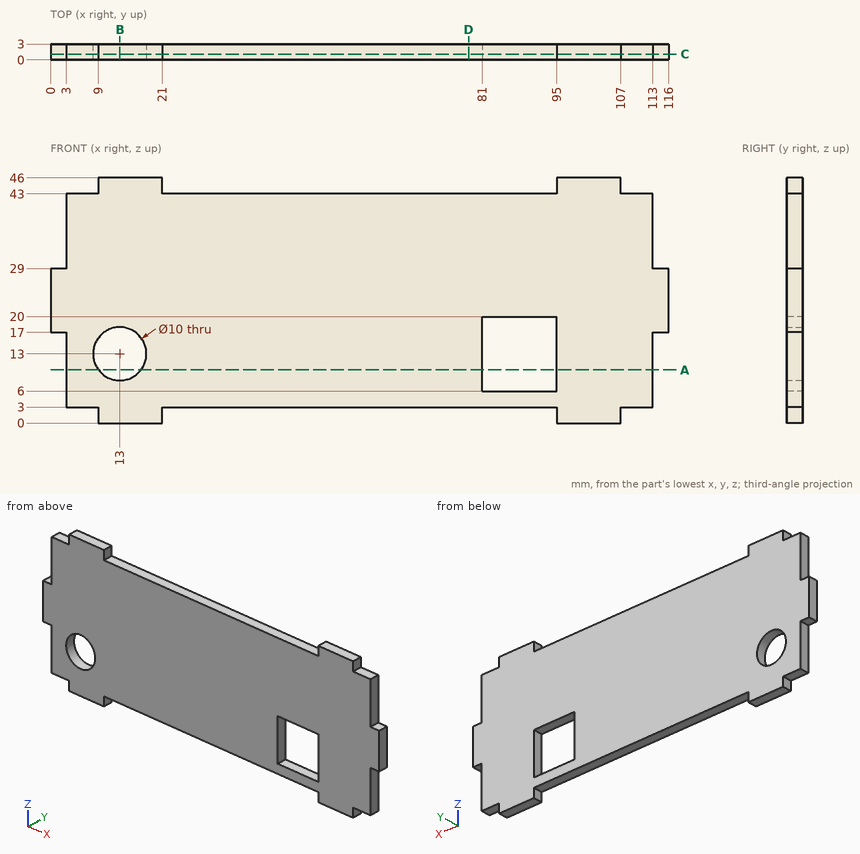
Can you work these out from the drawing? Everything is in mm from the part's minimum corner. Coordinates: 2 decimals unless noted, no trailing zeros. Loops run counter-clockwise (first coordinate to the right, second up) from the corner with the lowest first, then second, coordinate; pieces in that order, holes last. Notation, with made-up numbers: (3, 76.25) -> (10, 76.25) arc R31 ccw to (10, 101.25) -> close; hole circle Ø1 at (24, 83.5). An arc over 180 degrees is marked (long way). Return JSON: item names as keys, results as strings.
1) I need wall thicknesses on line 1 (X direction, y = 2.8, z = 19); line 2 (X direction, y = 2.15, z = 15); line 3 (Z direction, x = 13, y = 1.8). Which ranges of each line are inside material? Lowest first, please. Write a range as from..to.
Results below:
{"line 1": "0..81, 95..116", "line 2": "3..8.42, 17.58..81, 95..113", "line 3": "0..8, 18..46"}
2) If we section it at A-A, the plane z = 10: Write out the boundary of the cut face in (x, y), then the cut area to 3 significant figures.
Results below:
{"outline": "(3, 0) -> (9, 0) -> (9, 3) -> (3, 3) -> close; (17, 0) -> (81, 0) -> (81, 3) -> (17, 3) -> close; (95, 0) -> (113, 0) -> (113, 3) -> (95, 3) -> close", "area": "264 mm²"}
3) Will these pins go through, and if not, where does the flat tip stop? pin 1 (1 mm diameter, centred on x = 92, y = 2.5, fed in from +Z); pin 2 (1.5 mm diameter, centred on y = 2, z = 1, fed in from +X); pin 3 (1.5 mm diameter, centred on y = 2, z = 1, fed in from -X).
Results below:
{"pin 1": "z = 43", "pin 2": "x = 107", "pin 3": "x = 9"}
4) If we section it at C-C, the plane y = 1.1: Count the separate pieces of the cut face and the enclosed holes in it, then the cut area to 3 significant figures.
Results below:
{"separate pieces": "1", "enclosed holes": "2", "area": "4,340 mm²"}
5) If we section it at B-B, the plane x = 13: Write out the boundary of the cut face in (y, z), then the cut area to 3 significant figures.
Results below:
{"outline": "(0, 0) -> (3, 0) -> (3, 8) -> (0, 8) -> close; (0, 18) -> (3, 18) -> (3, 46) -> (0, 46) -> close", "area": "108 mm²"}
6) If we section it at D-D, the plane x = 78.5: Write out the boundary of the cut face in (y, z), then the cut area to 3 significant figures.
Results below:
{"outline": "(0, 3) -> (3, 3) -> (3, 43) -> (0, 43) -> close", "area": "120 mm²"}
